Here's how the part is built. I have some questions about the finished solid (model axes, mm). Coordinates: 2 decimals unless noted, no trailing zeros. Write each loop counter-clockwise with the first axis right and the second up, starting at its lowest first coordinate (ties: lowest second). Pieces come first, ordered by that corner, then holes. Notation, with made-up numbers: M 85,85.5 L 141,85.5 A10 ccw 141,92.5 Z; hole C 67.25,42.25 d5. An arc over 180 degrees is marked long. Use a Markdown table: item, result.
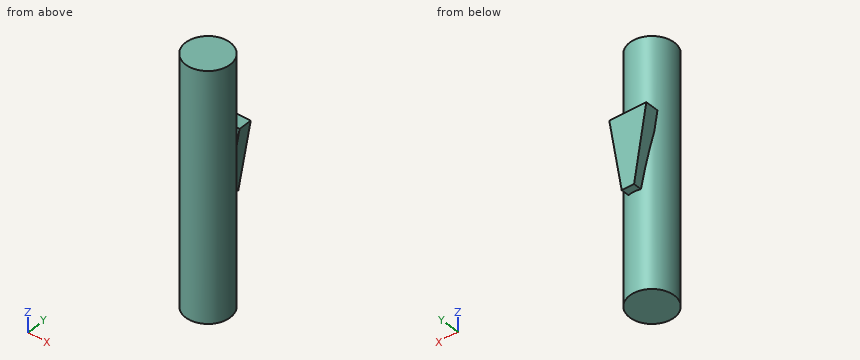
Autodesk Inventor part; units mm, degrees
ref_plane "Work Plane1" through (0, 9, 0) normal (0, 1, 0) x (-1, 0, 0)
ref_plane "YZ Plane" through (0, 0, 0) normal (1, 0, 0) x (0, 1, 0)
ref_plane "XY Plane" through (0, 0, 0) normal (0, 0, 1) x (1, 0, 0)
sketch "Sketch4" plane through (0, 0, 0) normal (0, 0, 1) x (1, 0, 0)
  circle A0 centre (0, 0) radius 9
  dimension "d5" = 18
sketch "Sketch5" plane through (0, 0, 0) normal (1, 0, 0) x (0, 1, 0)
  point P0 (0, 0)
ref_plane "Work Plane1" through (0, 9, 0) normal (0, 1, 0) x (-1, 0, 0)
sketch "Sketch6" plane through (0, 9, 0) normal (0, 1, 0) x (-1, 0, 0)
  line L0 (0, 0) -> (0, -100)
  line L1 (0, -30) -> (7.5, -30)
  line L2 (7.5, -30) -> (2.5456, -60)
  line L3 (2.5456, -60) -> (-2.4544, -60)
  line L4 (-2.4544, -60) -> (-7.5, -30)
  line L5 (-7.5, -30) -> (0, -30)
  dimension "d7" = 100
  dimension "d8" = 5
  dimension "d9" = 7.5
  dimension "d10" = 7.5
  dimension "d11" = 30
  dimension "d12" = 40
extrude "Extrusion3" add sketch "Sketch4" against normal blind 100
extrude "Extrusion4" add sketch "Sketch6" along normal blind 3 and the other way blind 2.5
1. Suppose I cut it at B-B on z = -87.5. Write out the boundary of the cut face in (x, y).
Answers follow:
| item | result |
|---|---|
| outline | C 0,0 d18 |
2. Suppose I cut it at A-A on x = 0. Write out the boundary of the cut face in (y, z).
Answers follow:
| item | result |
|---|---|
| outline | M -9,-100 L 9,-100 L 9,-60 L 12,-60 L 12,-30 L 9,-30 L 9,0 L -9,0 Z |
3. Suppose I cut it at D-D on z = -40. Write out the boundary of the cut face in (x, y).
Answers follow:
| item | result |
|---|---|
| outline | M -5.85,6.84 A9 ccw long 5.82,6.87 L 5.82,12 L -5.85,12 Z |
4. I need wall thicknesses on probe 1 along Y at (x, z) = (-6.5, -35); probe 2 along Y at (x, z) = (0.5, -32.5); probe 3 along X at (y, z) = (7, -52.5). Which ranges of each line are inside material? Lowest first, please.
Answers follow:
| item | result |
|---|---|
| probe 1 | y = -6.22 to 6.22, 6.5 to 12 |
| probe 2 | y = -8.99 to 12 |
| probe 3 | x = -5.66 to 5.66 |
5. Suppose I cut it at C-C on z = -50. Write out the boundary of the cut face in (x, y), and give its area (3 significant figures).
Answers follow:
| item | result |
|---|---|
| outline | M -4.2,7.96 A9 ccw long 4.14,7.99 L 4.14,12 L -4.2,12 Z |
| area | 282 mm2 |
6. Will these pins go through, and if not, where does the flat tip stop? pin 1 Ø1.5 at (x, y) = (-2.5, 3.5) entering from +Z; pin 2 Ø6 at (y, z) = (6.5, -82.5) entering from -X; pin 3 Ø1 at (x, z) = (7, -33) entering from -Y; pin 4 Ø8 at (y, z) = (-4.5, -18) entering from -X.
Answers follow:
| item | result |
|---|---|
| pin 1 | stops at z = 0 |
| pin 2 | stops at x = -8.29 |
| pin 3 | stops at y = -6.22 |
| pin 4 | stops at x = -8.99 |
